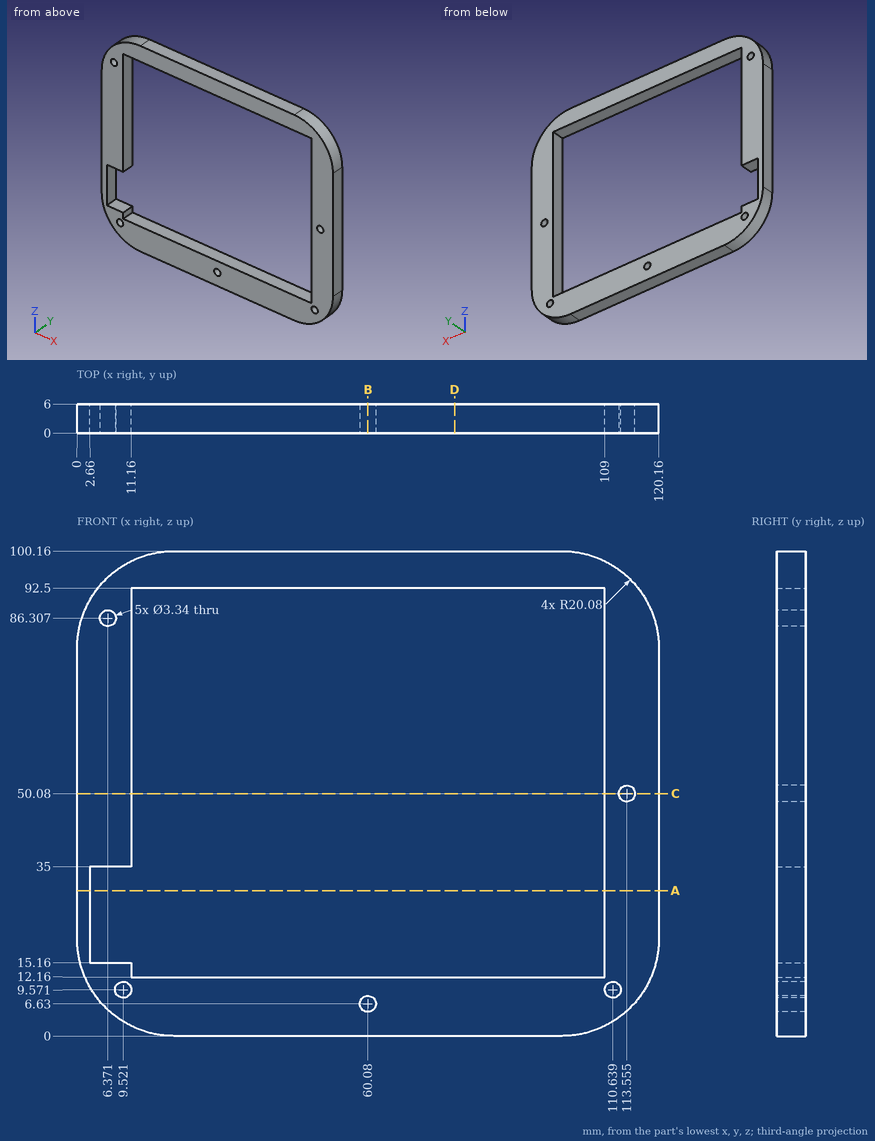
Source: three-view drawing plus pictorial views. Frame: mm from the lowest corner of the part. Coordinates: 2 decimals unless noted, no trailing zeros. Loops run counter-clockwise (first coordinate to the right, second up) from the corner with the lowest first, then second, coordinate; pieces in that order, holes last. Notation, with made-up numbers: (75, -3.75) -> (126, -3.75) arc R16 ccw to (126, 11.25) -> close; hole circle Ø1 at (-14, 55.25). An arc over 180 degrees is marked (long way). Answer in a Markdown table with one row per item. Add a question column.
Q1. Contact query for flat-ended pins moving along their axis: pin 1 Ø2 at (y, z) = (4.5, 18) entering from -X; pin 2 Ø2.5 at (y, z) = (3.5, 13) entering from +X (1 decimal); pin 3 Ø3 at (x, y) = (7.5, 3) entering from +Z (1 decimal). Output: stop coordinate, or through.
Q2. Ray query, line 1 along Z through (x, y) = (60.08, 3.6); line 2 along Z through (x, y) = (30, 3.2); line 3 along X through (y, z) = (2.4, 26). Return the intervals inside material, ascending.
Q3. Section A-A on z = 30. Return the cut outline in (x, y).
Q4. Section B-B on x = 60.08. Return the cut outline in (y, z).
Q5. Section C-C on z = 50.08. Return the cut outline in (x, y) (1 decimal), and give its area (3 significant figures).
Q6. Section D-D on x = 78. Return the cut outline in (y, z).
Computed values:
| question | item | result |
|---|---|---|
| 1 | pin 1 | stops at x = 0.03 |
| 1 | pin 2 | stops at x = 119.3 |
| 1 | pin 3 | stops at z = 96.8 |
| 2 | line 1 | z = 0 to 4.96, 8.3 to 12.16, 92.5 to 100.16 |
| 2 | line 2 | z = 0 to 12.16, 92.5 to 100.16 |
| 2 | line 3 | x = 0 to 2.66, 109 to 120.16 |
| 3 | outline | (0, 0) -> (2.66, 0) -> (2.66, 6) -> (0, 6) -> close; (109, 0) -> (120.16, 0) -> (120.16, 6) -> (109, 6) -> close |
| 4 | outline | (0, 0) -> (6, 0) -> (6, 4.96) -> (0, 4.96) -> close; (0, 8.3) -> (6, 8.3) -> (6, 12.16) -> (0, 12.16) -> close; (0, 92.5) -> (6, 92.5) -> (6, 100.16) -> (0, 100.16) -> close |
| 5 | outline | (0, 0) -> (11.2, 0) -> (11.2, 6) -> (0, 6) -> close; (109, 0) -> (111.9, 0) -> (111.9, 6) -> (109, 6) -> close; (115.2, 0) -> (120.2, 0) -> (120.2, 6) -> (115.2, 6) -> close |
| 5 | area | 114 mm^2 |
| 6 | outline | (0, 0) -> (6, 0) -> (6, 12.16) -> (0, 12.16) -> close; (0, 92.5) -> (6, 92.5) -> (6, 100.16) -> (0, 100.16) -> close |
